```python
from build123d import *

# Parameters (mm, degrees)
SKETCH2_R          = 2.75
CUT_EXTRUDE1_DEPTH = 0.1
CUT_EXTRUDE2_DEPTH = 0.1
FILLET1_R          = 0.5
SKETCH4_W          = 0.25
SKETCH4_H          = 2.5


with BuildPart() as part:
    # Sketch1 → Revolve1 (revolve)
    with BuildSketch(Plane.XY, mode=Mode.PRIVATE) as revolve1_sk:
        with BuildLine():
            Line((3.15, 15), (0, 15))
            Line((0, 15), (0, 0))
            Line((0, 0), (3.030208333, 0))
            ThreePointArc((3.030208333, 0), (3.115870139, 0.362697063), (3.030208333, 0.725394126))
            ThreePointArc((3.030208333, 0.725394126), (2.940770958, 0.972019442), (2.910416667, 1.232599004))
            Line((2.910416667, 1.232599004), (2.910416667, 1.642400996))
            ThreePointArc((2.910416667, 1.642400996), (2.941064683, 1.842850794), (3.030208333, 2.024984899))
            ThreePointArc((3.030208333, 2.024984899), (3.119351983, 2.207119004), (3.15, 2.407568802))
            Line((3.15, 2.407568802), (3.15, 15))
        make_face()
    revolve(revolve1_sk.sketch.rotate(Axis((0, 15, 0), (0, -1, 0)), 270), axis=Axis((0, 15, 0), (0, -1, 0)))

    # Sketch2 → Cut-Extrude1 (cut)
    with BuildSketch(Plane(origin=(0, 15, 0), x_dir=(-1, 0, 0), z_dir=(0, 1, 0))):
        with Locations(Location((0, 0, 0), (0, 0, 270))):
            Circle(SKETCH2_R)
    extrude(amount=-CUT_EXTRUDE1_DEPTH, mode=Mode.SUBTRACT)

    # Sketch3 → Cut-Extrude2 (cut)
    with BuildSketch(Plane(origin=(0, 14.9, 0), x_dir=(-1, 0, 0), z_dir=(0, 1, 0))):
        Polygon((1.653472744, -1.932293167), (1.837973446, -1.757720858), (0.142645036, 0.03402539), (0.846678598, 2.398095985), (0.603244193, 2.470592124), (-0.10078937, 0.10652153), (-2.500151342, -0.465802817), (-2.441217638, -0.712871266), (-0.041855666, -0.14054692), align=None)
    extrude(amount=-CUT_EXTRUDE2_DEPTH, mode=Mode.SUBTRACT)

    # Fillet1
    # the kernel refuses this fillet: 0.5 mm, written as the material it takes off along each edge
    with BuildSketch(Plane(origin=(0, 15, 0), x_dir=(0, 0, -1), z_dir=(-1, 0, 0))) as fillet1_piece_1:
        with BuildLine():
            CenterArc((2.65, 0.489897949), FILLET1_R, 281.536959033, 78.463040967)
            Line((3.15, 0.489897949), (3.16, 0.489897949))
            Line((3.16, 0.489897949), (3.16, 0))
            Line((3.16, 0), (3.15, -0.01))
            ThreePointArc((3.15, -0.01), (2.95, -0.01), (2.752, -0.009797959))
            Line((2.752, -0.009797959), (2.75, 0))
        make_face()
    revolve(axis=Axis((0, 15, 0), (0, -1, 0)), mode=Mode.SUBTRACT)
    with BuildSketch(Plane(origin=(0, 0, 0), x_dir=(0, 0, -1), z_dir=(-1, 0, 0))) as fillet1_piece_2:
        with BuildLine():
            CenterArc((2.583882439, -0.5), FILLET1_R, 333.771257748, 116.228742252)
            Line((2.583882439, 0), (2.583882439, 0.01))
            Line((2.583882439, 0.01), (3.030208333, 0.01))
            Line((3.030208333, 0.01), (3.039151656, 0.004474035))
            ThreePointArc((3.039151656, 0.004474035), (3.125866344, -0.360201414), (3.041371195, -0.725397511))
            Line((3.041371195, -0.725397511), (3.032400827, -0.720977952))
        make_face()
    revolve(axis=Axis((0, 0, 0), (0, -1, 0)), mode=Mode.SUBTRACT)

    # Sketch4 → Revolve2 (revolve)
    with BuildSketch(Plane(origin=(0, 0, 0), x_dir=(-1, 0, 0), z_dir=(0, 0, -1)), mode=Mode.PRIVATE) as revolve2_sk:
        with Locations((-1.375, -1.25)):
            Rectangle(SKETCH4_W, SKETCH4_H)
    revolve2 = revolve(revolve2_sk.sketch.rotate(Axis((1.25, -2.5, 0), (0, 1, 0)), 180), axis=Axis((1.25, -2.5, 0), (0, 1, 0)))

    # Simetría2: Revolve2 across plane
    add(revolve2.mirror(Plane(origin=(0, 0, 0), x_dir=(0, 0, 1), z_dir=(1, 0, 0))))


solid = part.part
```
For this review, take the finished solid that the model builds, in its own axes (mm). Round coordinates to 2 decimals unless told otherwise and drop trailing zeros. Order: outer loops, then holes, each group sorted by start corner. A loop starts at its lowest first (then second) coordinate and runs counter-clockwise, first axis right, second up. Notation, with made-up numbers: (22.25, 5.5) -> (63.25, 5.5) arc R27 cw to (63.25, 38.5) -> close; hole circle Ø4 at (17.5, 69). An arc over 180 degrees is marked (long way). Use a Markdown table: item, result.
Item 1: For line 1 along Y through (x, z) = (0.75, 0.75); line 2 along Y through (x, z) = (-0.5, 2); line 3 along Z through (x, y) = (-1, 8.25), list the stretches that pass through material, from the lowest coordinate up. Write a range as [from, to].
Resolved:
| item | result |
|---|---|
| line 1 | y = [0, 14.9] |
| line 2 | y = [0, 14.8] |
| line 3 | z = [-2.99, 2.99] |
Item 2: For pin 1 (1 mm diameter, centred on y = 6, z = -1.5, fed in from +X); pin 2 (3 mm diameter, centred on x = 0.5, z = 1, fed in from +Y); pin 3 (1 mm diameter, centred on x = 1, y = 9, fed in from +Z); pin 4 (2 mm diameter, centred on x = 1, z = -2.5, fed in from +Y), all flat-tipped, find the tip position at first contact; note any pin that passes through.
Resolved:
| item | result |
|---|---|
| pin 1 | stops at x = 2.99 |
| pin 2 | stops at y = 14.9 |
| pin 3 | stops at z = 3.11 |
| pin 4 | stops at y = 15 |
Item 3: Draft analysis for pull direction X (two halves, no side actions). For faces 1 (the cylindrical face through (-1.917, 8.544, 2.5)), 2 (the flat face through (0, 14.9, -1)), state which applies: +X half, -X half, draft (parallel to the pull), parting line (faces both ways), or undercut.
Resolved:
| item | result |
|---|---|
| face 1 | parting line |
| face 2 | undercut |
Item 4: Take a section at A-A (y = 9.75). State the section outline as (x, z) points, plus the area to 3 significant figures.
Resolved:
| item | result |
|---|---|
| outline | circle Ø6.3 at (0, 0) |
| area | 31.2 mm² |
